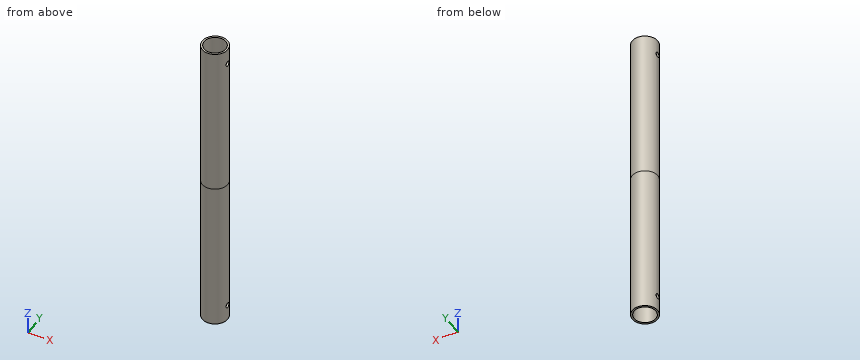
```python
from build123d import *

# Parameters (mm, degrees)
SKETCH1_R           = 10
SKETCH1_R_2         = 8.5
BOSS_EXTRUDE1_DEPTH = 120
SKETCH2_R           = 2
CUT_EXTRUDE1_DEPTH  = 121.830459736


with BuildPart() as part:
    # Sketch1 → Boss-Extrude1 (new body)
    with BuildSketch(Plane.XY):
        Circle(SKETCH1_R)
        Circle(SKETCH1_R_2, mode=Mode.SUBTRACT)
    boss_extrude1 = extrude(amount=BOSS_EXTRUDE1_DEPTH)

    # Sketch2 → Cut-Extrude1 (cut, symmetric)
    with BuildSketch(Plane(origin=(0, 0, 0), x_dir=(0, 0, -1), z_dir=(1, 0, 0))):
        with Locations((-107.5, 0)):
            Circle(SKETCH2_R)
    cut_extrude1 = extrude(amount=CUT_EXTRUDE1_DEPTH, both=True, mode=Mode.SUBTRACT)

    # Mirror1: Boss-Extrude1, Cut-Extrude1 across plane
    add(boss_extrude1.mirror(Plane.XY))
    add(cut_extrude1.mirror(Plane.XY), mode=Mode.SUBTRACT)


solid = part.part
```
Input: part model. Units: mm. Frame: model coordinates. Give positions to 0.01 mm unless a question says otherwise; leave off trailing zeros. Order: outer loops, then holes, each group sorted by start corner. A loop starts at its lowest first (then second) coordinate and runs counter-clockwise, first axis right, second up. Notation, with made-up numbers: (74, -13.5) - (85, -13.5) arc R31 ccw to (85, 24.5) - close; hole circle Ø4 at (-39, 82). An arc over 180 degrees is marked (long way). Use a Markdown table: item, result.
(1) Section query A-A (x = 0). Output: boundary loops of the cut face in (y, z).
Computed values:
| item | result |
|---|---|
| outline | (-10, -120) - (-8.5, -120) - (-8.5, 120) - (-10, 120) - close; (8.5, -120) - (10, -120) - (10, 120) - (8.5, 120) - close |
(2) Pin query (flat end, axial travel): pin 1 (10 mm diameter, centred on x = 0, y = 0, fed in from +Z); pin 2 (2 mm diameter, centred on x = 1.5, z = -93.5, fed in from +Y); pin 3 (3 mm diameter, centred on x = 4, z = -38, fed in from +Y); pin 4 (1 mm diameter, centred on y = -7, z = -3.5, fed in from +X). Return the tip coordinate at first contact, or that it passes through.
Computed values:
| item | result |
|---|---|
| pin 1 | passes through |
| pin 2 | stops at y = 9.99 |
| pin 3 | stops at y = 9.68 |
| pin 4 | stops at x = 7.6 |
(3) Section query C-C (z = -107.5). Output: boundary loops of the cut face in (x, y), then the cut area to 3 significant figures.
Computed values:
| item | result |
|---|---|
| outline | (-9.8, -2) arc R10 ccw to (9.8, -2) - (8.26, -2) arc R8.5 cw to (-8.26, -2) - close; (-9.8, 2) - (-8.26, 2) arc R8.5 cw to (8.26, 2) - (9.8, 2) arc R10 ccw to start |
| area | 75.1 mm2 |
(4) Section query D-D (z = 30). Output: boundary loops of the cut face in (x, y).
Computed values:
| item | result |
|---|---|
| outline | circle Ø20 at (0, 0); hole circle Ø17 at (0, 0) |
(5) Section query B-B (y = 0). Output: boundary loops of the cut face in (x, z), then the cut area to 3 significant figures.
Computed values:
| item | result |
|---|---|
| outline | (-10, -120) - (-8.5, -120) - (-8.5, -109.5) - (-10, -109.5) - close; (-10, -105.5) - (-8.5, -105.5) - (-8.5, 105.5) - (-10, 105.5) - close; (-10, 109.5) - (-8.5, 109.5) - (-8.5, 120) - (-10, 120) - close; (8.5, -120) - (10, -120) - (10, -109.5) - (8.5, -109.5) - close; (8.5, -105.5) - (10, -105.5) - (10, 105.5) - (8.5, 105.5) - close; (8.5, 109.5) - (10, 109.5) - (10, 120) - (8.5, 120) - close |
| area | 696 mm2 |
(6) Line query: line 1 (Z direction, x = 8.6, y = 0); line 2 (Y direction, x = 0, z = 36.5). Output: solid intervals per line, ascending. Write a range as from..to.
Computed values:
| item | result |
|---|---|
| line 1 | z = -120..-109.5, -105.5..105.5, 109.5..120 |
| line 2 | y = -10..-8.5, 8.5..10 |
